Source: CAD feature listing. Evaluate the final solid. Frame: model axes, mm. A direction names the side the tool comes from. Give positions to 0.01 mm unless a question says otherwise; leave off trailing zeros. Loops run counter-clockwise (first coordinate to the right, second up) from the corner with the lowest first, then second, coordinate; pieces in that order, holes last.
Autodesk Inventor part; units mm, degrees
ref_plane "YZ Plane" through (0, 0, 0) normal (1, 0, 0) x (0, 1, 0)
ref_plane "XZ Plane" through (0, 0, 0) normal (0, 1, 0) x (-1, 0, 0)
ref_plane "XY Plane" through (0, 0, 0) normal (0, 0, 1) x (1, 0, 0)
sketch "Эскиз1" plane through (0, 0, 0) normal (1, 0, 0) x (0, 1, 0)
  line L0 (-14, 0) -> (14, 0)
  line L1 (0, -56) -> (0, 56)
  line L2 (10, 40) -> (-10, 40)
  line L3 (-10, 40) -> (-10, -40)
  line L4 (-10, -40) -> (10, -40)
  line L5 (10, -40) -> (10, 40)
  point P0 (0, 0)
  dimension "d0" = 20
  dimension "d1" = 10
  dimension "d2" = 80
  dimension "d3" = 40
extrude "Выдавливание1" add sketch "Эскиз1" against normal blind 70
fillet "Сопряжение1" radius 5 2 edges at (0, 0, 40) (0, 0, -40)
chamfer "Фаска1" distance 1 angle 45 10 edges at (-37.5, 10, 40) (-1.4645, 10, 38.5355) (0, 10, 0) (-1.4645, 10, -38.5355) (-37.5, 10, -40) (-37.5, -10, 40) (-1.4645, -10, 38.5355) (0, -10, 0) (-1.4645, -10, -38.5355) (-37.5, -10, -40)
chamfer "Фаска2" distance 1 angle 45 4 edges at (-70, 10, 0) (-70, 0, 40) (-70, -10, 0) (-70, 0, -40)
sketch "Эскиз3" plane through (-70, 0, 0) normal (-1, 0, 0) x (0, 0, 1)
  line L0 (-56, 0) -> (56, 0)
  line L1 (0, 14) -> (0, -14)
  circle A0 centre (14, 0) radius 3
  circle A1 centre (-14, 0) radius 3
  dimension "d42" = 6
  dimension "d43" = 6
  dimension "d44" = 28
  dimension "d45" = 14
hole "Отверстие2" at (-70, 0, 14) at (-70, 0, -14) direction (1, 0, 0) diameter 6 depth 10 tip angle 118 countersink diameter 8 countersink angle 45
sketch "Эскиз4" plane through (-70, 0, 0) normal (-1, 0, 0) x (0, 0, 1)
  line L0 (0, 14) -> (0, -14)
  line L1 (-56, 0) -> (56, 0)
  circle A0 centre (25, 0) radius 5
  circle A1 centre (-25, 0) radius 5
  point P0 (0, 0)
  dimension "d46" = 10
  dimension "d47" = 50
  dimension "d48" = 25
hole "Отверстие3" at (-70, 0, 25) at (-70, 0, -25) direction (1, 0, 0) diameter 8.376 depth 31.3 tip angle 118 countersink diameter 13.2 countersink angle 90
sketch "Эскиз6" plane through (0, 0, 0) normal (0, 1, 0) x (-1, 0, 0)
  line L0 (-14, 0) -> (84, 0)
  line L1 (0, -56) -> (0, 56)
  line L2 (70, -39) -> (70, 39)
  line L3 (15, 7.5) -> (15, -7.5) construction
  arc A0 (21, 7.5) -> (9, 7.5) centre (15, 7.5) ccw
  arc A1 (9, -7.5) -> (21, -7.5) centre (15, -7.5) ccw
  line L4 (21, 7.5) -> (21, -7.5)
  line L5 (9, 7.5) -> (9, -7.5)
  point P0 (0, 0)
  dimension "d56" = 12
  dimension "d57" = 15
  dimension "d58" = 7.5
  dimension "d59" = 55
extrude "Выдавливание2" cut sketch "Эскиз6" along normal through all both and the other way through all
chamfer "Фаска4" distance 0.2 angle 45 8 edges at (-9, -10, 0) (-15, -10, -13.5) (-21, -10, 0) (-15, -10, 13.5) (-21, 10, 0) (-15, 10, -13.5) (-9, 10, 0) (-15, 10, 13.5)
properties part number "ОПОРА_02"
(1) Ray query, line 1 along Z through (x, y) = (-15.5, -3.5); line 2 along Y through (x, z) = (-63.25, 14); line 3 along X through (y, z) = (7.75, 6.5). Return the intervals inside material, ascending.
A:
line 1: z = -40 to -13.48, 13.48 to 40
line 2: y = -10 to -3, 3 to 10
line 3: x = -70 to -21, -9 to 0
(2) Section B-B, the plane z = -2. Return the cut outline in (x, y).
A:
outline: (-70, -9) - (-69, -10) - (-21.2, -10) - (-21, -9.8) - (-21, 9.8) - (-21.2, 10) - (-69, 10) - (-70, 9) - close; (-9, -9.8) - (-8.8, -10) - (-1, -10) - (0, -9) - (0, 9) - (-1, 10) - (-8.8, 10) - (-9, 9.8) - close
(3) Reachability of faces 5 (the flat face through (-35, 10, -1)), 6 (the cylindrical face through (-15.1, -0.1, -13.5)), 7 (the cylindrical face through (-64, 0, 11)) from +Z, -Z, +X, -X, +Y, -Y: full face, straight path, thin tool, end or side. Return the list, or none.
A:
face 5: +Z, -Z, +X, -X, +Y
face 6: +Y, -Y
face 7: -X
(4) Section A-A, the plane x = -42. Return the cut outline in (y, z).
A:
outline: (-10, -39) - (-9, -40) - (9, -40) - (10, -39) - (10, 39) - (9, 40) - (-9, 40) - (-10, 39) - close; hole circle Ø8.38 at (0, -25); hole circle Ø8.38 at (0, 25)
(5) Mould query, pull axis X, two halves, no side actions, for faces 1 (the conical face through (-67.737, 0.92, 16.921)), 2 (the flat face through (-37, 0, -40)), 3 (the cylindrical face through (-14.9, -0.1, 13.5)), 4 (the flat face through (-9, 0, 0)). Classes: pulls with the +X half, pulls with the -X half, needs draft (parallel to the pull), parting line crosses it, or undercut.
A:
face 1: pulls with the -X half
face 2: needs draft
face 3: undercut
face 4: undercut
(6) First-contact query: pin 1 (7.5 mm diameter, centred on y = 0, z = -25, fed in from -X); pin 2 (5.5 mm diameter, centred on y = 0, z = -14, fed in from -X). Flat tips, straight axial feed; report the tip coordinate or a pass-through.
A:
pin 1: stops at x = -38.44
pin 2: stops at x = -59.85
